from build123d import *

# Parameters (mm, degrees)
EXTRUDE2_DEPTH = 13
EXTRUDE3_REACH = 74.426
SKETCH2_R      = 4
SKETCH3_R      = 4
EXTRUDE4_DEPTH = 73.426406871
SKETCH4_W      = 18
SKETCH4_H      = 8
EXTRUDE5_DEPTH = 13
FILLET1_R      = 5


with BuildPart() as part:
    # Sketch1 → Extrude2 (new body)
    with BuildSketch(Plane(origin=(0, 0, 0), x_dir=(1, 0, 0), z_dir=(0, 1, 0))):
        Polygon((15, -36.213203436), (36.213203436, -15), (36.213203436, 15), (15, 36.213203436), (-15, 36.213203436), (-36.213203436, 15), (-36.213203436, -15), (-15, -36.213203436), align=None)
    extrude(amount=EXTRUDE2_DEPTH)

    # Sketch2 → Extrude3 (cut, up to next)
    with BuildSketch(Plane(origin=(36.213203436, 0, 0), x_dir=(0, 0, -1), z_dir=(1, 0, 0)), mode=Mode.PRIVATE) as extrude3_sk1:
        with Locations((0, 6.5)):
            Circle(SKETCH2_R)
    extrude3_tool1 = extrude(extrude3_sk1.sketch, amount=-EXTRUDE3_REACH, mode=Mode.PRIVATE) & part.part
    add(extrude3_tool1.solids().sort_by_distance((36.213203, 6.5, 0))[0], mode=Mode.SUBTRACT)

    # Sketch3 → Extrude4 (cut, through all)
    with BuildSketch(Plane.XY.offset(36.213203436)):
        with Locations((0, 6.5)):
            Circle(SKETCH3_R)
    extrude(amount=-EXTRUDE4_DEPTH, mode=Mode.SUBTRACT)

    # Sketch4 → Extrude5 (cut)
    with BuildSketch(Plane(origin=(0, 13, 0), x_dir=(1, 0, 0), z_dir=(0, 1, 0))):
        with Locations((0, -14)):
            Rectangle(SKETCH4_W, SKETCH4_H)
        with Locations((0, 14)):
            Rectangle(SKETCH4_W, SKETCH4_H)
    extrude(amount=-EXTRUDE5_DEPTH, mode=Mode.SUBTRACT)

    # Fillet1
    fillet1_edges = [part.edges().sort_by_distance(p)[0] for p in [
        (36.213203436, 6.5, 15),
        (15, 6.5, 36.213203436),
        (-15, 6.5, 36.213203436),
        (-36.213203436, 6.5, 15),
        (-36.213203436, 6.5, -15),
        (-15, 6.5, -36.213203436),
        (15, 6.5, -36.213203436),
        (36.213203436, 6.5, -15),
    ]]
    fillet(fillet1_edges, radius=FILLET1_R)


solid = part.part
For this review, take the finished solid that the model builds, in its own axes (mm). A direction names the side the tool comes from. Round coordinates to 2 decimals unless told otherwise and drop trailing zeros. Loops run counter-clockwise (first coordinate to the right, second up) from the corner with the lowest first, then second, coordinate; pieces in that order, holes last. Notation, with made-up numbers: (30, 31) - (76, 31) arc R8 ccw to (76, 42) - close; hole circle Ø6 at (-32.5, 18). An arc over 180 degrees is marked (long way). Put each result on its own line as item: value. Start each with the question number.
1. Consider section D-D on x = -24. State the section outline as (y, z) points.
2. For faces 1 (the cylindrical face through (-14.82, 6.59, -35.84)), 2 (the flat face through (-4, 8, -18)), list the 3-axis set-ups (+Z, -Z, +X, -X, +Y, -Y) from which the entire face can be reached by the end or side of a thin tool; tool diameter is ignored.
3. Consider section C-C on y = 6.5. State how many separate pieces and enclosed holes the cut face has, plus the area to 3 significant figures.
4. For probe 1 along Y at (x, z) = (-24.5, 0); probe 2 along X at (y, z) = (6.5, -5.75); probe 3 along Z at (x, y) = (8, 3.5), list the stretches that pass through material, from the lowest coordinate up. Write a range as [from, to].
5. Consider section B-B on z = 8. State the section outline as (x, y) points, plus the area to 3 significant figures.
6. Consider section A-A on x = 5. State the section outline as (y, z) points, plus the area to 3 significant figures.
7. Mouldability with a two-part tool opening along X and no side actions: class faces 3 (the flat face through (3.1, 3.5, -36.213)), 4 (the flat face through (-9, 7, -14)), 5 (the cylindrical face through (-0.867, 2.595, -26.979)), 6 (the flat face through (25.479, 6.409, 25.735)) as +X half, -X half, draft (parallel to the pull), parting line (faces both ways), or undercut.
8. Insertion check: P1, Ø6, axis at y = 7.5, z = 25.5, coming from the +X side; P2, Ø4, axis at y = 8, z = 26.5, coming from the +X side; P3, Ø2.5, axis at y = 4, z = 16, coming from the -X side. Each pin has a flat end and moves straight along its axis. Give the tip position at first contact, or say it passes through.
Result sheet:
1. outline: (0, -27.21) - (13, -27.21) - (13, 27.21) - (0, 27.21) - close; hole circle Ø8 at (6.5, 0)
2. face 1: -Z, -X, +Y, -Y
2. face 2: +Y, -Y
3. separate pieces: 4
3. enclosed holes: 0
3. area: 3,090 mm^2
4. probe 1: [0, 2.5], [10.5, 13]
4. probe 2: [-36.21, -4], [4, 36.21]
4. probe 3: [-36.21, -18], [-10, -2.65], [2.65, 10], [18, 36.21]
5. outline: (-36.21, 0) - (36.21, 0) - (36.21, 13) - (-36.21, 13) - close; hole circle Ø8 at (0, 6.5)
5. area: 891 mm^2
6. outline: (0, -36.21) - (13, -36.21) - (13, -18) - (0, -18) - close; (0, -10) - (13, -10) - (13, 10) - (0, 10) - close; (0, 18) - (13, 18) - (13, 36.21) - (0, 36.21) - close; hole circle Ø8 at (6.5, 0)
6. area: 683 mm^2
7. face 3: draft
7. face 4: undercut
7. face 5: undercut
7. face 6: +X half
8. P1: x = 28.71
8. P2: x = 26.71
8. P3: x = -35.87
